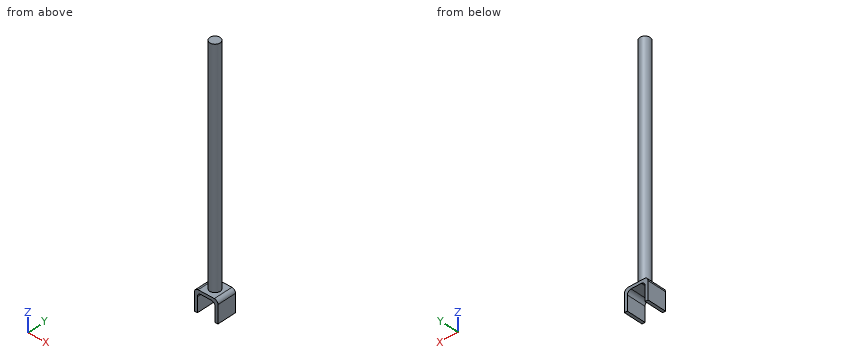
from build123d import *

# Parameters (mm, degrees)
BOSS_EXTRUDE1_DEPTH      = 13
BOSS_EXTRUDE1_DEPTH_BACK = 13
SKETCH2_R                = 7
BOSS_EXTRUDE2_DEPTH      = 307.5


with BuildPart() as part:
    # Sketch1 → Boss-Extrude1 (new, two sides: drawn at the far end of the back side and taken through both)
    with BuildSketch(Plane(origin=(0, 0, 0), x_dir=(1, 0, 0), z_dir=(0, 1, 0)).offset(-BOSS_EXTRUDE1_DEPTH_BACK)):
        with BuildLine():
            Line((7, -20.776256957), (-7, -20.776256957))
            ThreePointArc((-7, -20.776256957), (-10.535533906, -19.311790863), (-12, -15.776256957))
            Line((-12, -15.776256957), (-12, 4.223743043))
            Line((-12, 4.223743043), (-16, 4.223743043))
            Line((-16, 4.223743043), (-16, -19.776256957))
            ThreePointArc((-16, -19.776256957), (-14.535533906, -23.311790863), (-11, -24.776256957))
            Line((-11, -24.776256957), (11, -24.776256957))
            ThreePointArc((11, -24.776256957), (14.535533906, -23.311790863), (16, -19.776256957))
            Line((16, -19.776256957), (16, 4.223743043))
            Line((16, 4.223743043), (12, 4.223743043))
            Line((12, 4.223743043), (12, -15.776256957))
            ThreePointArc((12, -15.776256957), (10.535533906, -19.311790863), (7, -20.776256957))
        make_face()
    extrude(amount=BOSS_EXTRUDE1_DEPTH + BOSS_EXTRUDE1_DEPTH_BACK)

    # Sketch2 → Boss-Extrude2 (add)
    with BuildSketch(Plane.XY.offset(24.776256957)):
        Circle(SKETCH2_R)
    extrude(amount=BOSS_EXTRUDE2_DEPTH)


solid = part.part
For this review, take the finished solid that the model builds, in its own axes (mm). Round coordinates to 2 decimals unless told otherwise and drop trailing zeros. Order: outer loops, then holes, each group sorted by start corner. A loop starts at its lowest first (then second) coordinate and runs counter-clockwise, first axis right, second up. Notation, with made-up numbers: (37.5, 26) -> (53.5, 26) arc R22 cw to (53.5, 61) -> close; hole circle Ø1 at (67.5, 0). An arc over 180 degrees is marked (long way). Put each result on its own line as item: value.
Q1. Add section A-A on x = 0. Write out the cut boundary in (y, z), plus the area to 3 significant figures.
Check result:
outline: (-13, 20.78) -> (13, 20.78) -> (13, 24.78) -> (7, 24.78) -> (7, 332.28) -> (-7, 332.28) -> (-7, 24.78) -> (-13, 24.78) -> close
area: 4,410 mm2
Q2. Insertion check: pin 1 Ø4 at (x, z) = (-0.5, 293.5) entering from +Y; pin 2 Ø10 at (x, y) = (3, 3) entering from -Z; pin 3 Ø5 at (x, z) = (8, 294) entering from -Y. Each pin has a flat end and moves straight along its axis. Give the tip position at first contact, or say it passes through.
Check result:
pin 1: y = 7
pin 2: z = 20.68
pin 3: y = -4.33
Q3. For probe 1 along Z at (x, y) = (6, -1.5); probe 2 along Z at (x, y) = (5.5, -10.5); probe 3 along Y at (x, z) = (0, 251), list the stretches that pass through material, from the lowest coordinate up. Write a range as [from, to].
Check result:
probe 1: [20.78, 332.28]
probe 2: [20.78, 24.78]
probe 3: [-7, 7]
Q4. Add section B-B on y = 0. Write out the cut boundary in (x, z).
Check result:
outline: (-16, -4.22) -> (-12, -4.22) -> (-12, 15.78) arc R5 cw to (-7, 20.78) -> (7, 20.78) arc R5 cw to (12, 15.78) -> (12, -4.22) -> (16, -4.22) -> (16, 19.78) arc R5 ccw to (11, 24.78) -> (7, 24.78) -> (7, 332.28) -> (-7, 332.28) -> (-7, 24.78) -> (-11, 24.78) arc R5 ccw to (-16, 19.78) -> close
Q5. Add section C-C on z = 114.5. Write out the cut boundary in (x, y).
Check result:
outline: circle Ø14 at (0, 0)
